Could you check a few things on this model? Use its own coordinates, in mm. Round coordinates to 2 decimals unless told otherwise and drop trailing zeros. Loops run counter-clockwise (first coordinate to the right, second up) from the corner with the lowest first, then second, coordinate; pieces in that order, holes last. Notation, with made-up numbers: (28, 24) -> (39, 24) arc R16 ccw to (39, 48) -> close; hole circle Ø7 at (19, 38). An arc over 180 degrees is marked (long way). Write each question's results on one line, items separated by ' | '.
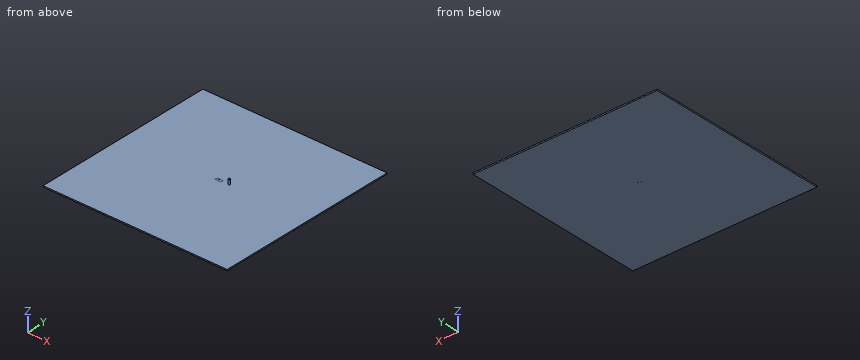
from build123d import *

# Parameters (mm, degrees)
F0_W     = 300
F0_H     = 300
F1_DEPTH = 2
F2_W     = 10
F2_H     = 4
F3_DEPTH = 0.1
F4_W     = 0.3
F4_H     = 0.3
F5_DEPTH = 3
F6_R     = 1.5
F7_DEPTH = 10


with BuildPart() as f1:
    # F0 (on Top) → F1 (new body)
    with BuildSketch(Plane.XY):
        Rectangle(F0_W, F0_H)
    extrude(amount=F1_DEPTH)

    # F2 (on face) → F3 (cut)
    with BuildSketch(Plane.XY.offset(2)):
        with Locations((5, 2)):
            Rectangle(F2_W, F2_H)
    extrude(amount=-F3_DEPTH, mode=Mode.SUBTRACT)

    # F4 (on face) → F5 (cut)
    with BuildSketch(Plane.XY.offset(2)):
        with Locations((1.15, 3.15)):
            Rectangle(F4_W, F4_H)
        with Locations((1.15, 1.15)):
            Rectangle(F4_W, F4_H)
        with Locations((3.15, 3.15)):
            Rectangle(F4_W, F4_H)
        with Locations((3.15, 1.15)):
            Rectangle(F4_W, F4_H)
        with Locations((5.15, 3.15)):
            Rectangle(F4_W, F4_H)
        with Locations((5.15, 1.15)):
            Rectangle(F4_W, F4_H)
        with Locations((7.15, 3.15)):
            Rectangle(F4_W, F4_H)
        with Locations((7.15, 1.15)):
            Rectangle(F4_W, F4_H)
        with Locations((9.15, 3.15)):
            Rectangle(F4_W, F4_H)
        with Locations((9.15, 1.15)):
            Rectangle(F4_W, F4_H)
    extrude(amount=-F5_DEPTH, mode=Mode.SUBTRACT)

    # F6 (on Top) → F7 (join)
    with BuildSketch(Plane.XY):
        with Locations((21, 2.5)):
            Circle(F6_R)
    extrude(amount=F7_DEPTH)


solid = f1.part
1) I want a section at A-A, the plane z = 4.25. Write out the boundary of the cut face in (x, y), plus the area to 3 significant figures.
Model answer:
outline: circle Ø3 at (21, 2.5) | area: 7.07 mm2
2) I need wall thicknesses on line 1 (Z direction, x = -62.5, y = 4). Which ranges of the line are inside material? Lowest first, please.
Model answer:
line 1: z = 0 to 2
3) I'm going to push a flat-ended pin straight in: pin 1 (5 mm diameter, centred on x = -41.5, y = 40.5, fed in from +Z). Where does the tip first touch, or does it pass through?
Model answer:
pin 1: stops at z = 2
4) I want a section at B-B, the plane y = 127. Write out the boundary of the cut face in (x, z), plus the area to 3 significant figures.
Model answer:
outline: (-150, 0) -> (150, 0) -> (150, 2) -> (-150, 2) -> close | area: 600 mm2
